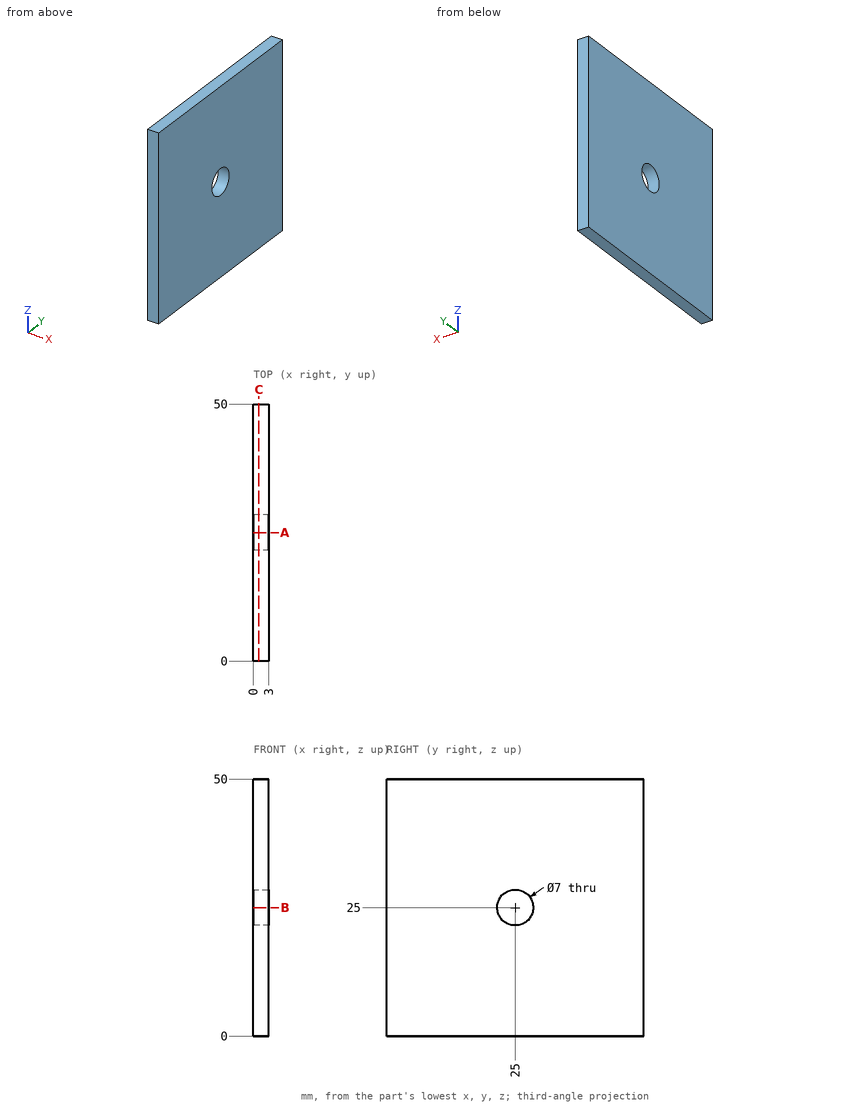
Answer from the drawing. Dimensions are ordinates in mm from the lowest x, y and z of the part. Round coordinates to 2 decimals unless told otherwise and drop trailing zeros. Loops run counter-clockwise (first coordinate to the right, second up) from the corner with the lowest first, then second, coordinate; pieces in that order, holes last. Notation, with made-up numbers: (17, 80.5) - (56, 80.5) arc R13 ccw to (56, 89.5) - close; hole circle Ø6 at (83.25, -21). An arc over 180 degrees is marked (long way). One line per item, written item: value.
Q1. Find section A-A on y = 25. Give the vertices of the cut face in (x, z), and give its area (3 significant figures).
Check values:
outline: (0, 0) - (3, 0) - (3, 21.5) - (0, 21.5) - close; (0, 28.5) - (3, 28.5) - (3, 50) - (0, 50) - close
area: 129 mm2
Q2. A straight line is drawn through the part: probe 1 along Y at (x, z) = (1.1, 25). Find the intervals that lie inside material, in ascending order.
Check values:
probe 1: 0 to 21.5, 28.5 to 50
Q3. Find section C-C on x = 1.1. Give the vertices of the cut face in (y, z), and give its area (3 significant figures).
Check values:
outline: (0, 0) - (50, 0) - (50, 50) - (0, 50) - close; hole circle Ø7 at (25, 25)
area: 2,460 mm2
Q4. This flat-tipped pin is pushed along its axis until it touches: pin 1 Ø5.5 at (y, z) = (25, 25) entering from -X. Where does it stop, or does it pass through?
Check values:
pin 1: through
